Geometry check sheet. Reference: the model listing, model coordinates, mm. A direction names the side the tool comes from. Give positions to 0.01 mm unless a question says otherwise; leave off trailing zeros. Loops run counter-clockwise (first coordinate to the right, second up) from the corner with the lowest first, then second, coordinate; pieces in that order, holes last.
```python
from build123d import *

# Parameters (mm, degrees)
SKETCH_1_R          = 80
SKETCH_1_R_2        = 60
EXTRUDE_1_DEPTH     = 80
CUT_EXTRUDE_1_DEPTH = 139.564064606
CUT_EXTRUDE_2_DEPTH = 139.564064606
SKETCH_4_R          = 20
SKETCH_4_R_2        = 7.5
EXTRUDE_2_DEPTH     = 80
FILLET_1_R          = 10


with BuildPart() as part:
    # 草图1 → 凸台-拉伸1 (new body)
    with BuildSketch(Plane.XY):
        Circle(SKETCH_1_R)
        Circle(SKETCH_1_R_2, mode=Mode.SUBTRACT)
    extrude(amount=EXTRUDE_1_DEPTH)

    # 草图2 → 切除-拉伸1 (cut, through all)
    with BuildSketch(Plane.XY.offset(80)):
        Polygon((60.621778265, 30.265727793), (64.721778265, 32.632863896), (64.721778265, 37.367136104), (60.621778265, 39.734272207), (56.521778265, 37.367136104), (56.521778265, 32.632863896), align=None)
        Polygon((4.1, 67.632863896), (4.1, 72.367136104), (0, 74.734272207), (-4.1, 72.367136104), (-4.1, 67.632863896), (0, 65.265727793), align=None)
        Polygon((56.521778265, -37.367136104), (60.621778265, -39.734272207), (64.721778265, -37.367136104), (64.721778265, -32.632863896), (60.621778265, -30.265727793), (56.521778265, -32.632863896), align=None)
        Polygon((-4.1, -67.632863896), (-4.1, -72.367136104), (0, -74.734272207), (4.1, -72.367136104), (4.1, -67.632863896), (0, -65.265727793), align=None)
        Polygon((-60.621778265, -30.265727793), (-64.721778265, -32.632863896), (-64.721778265, -37.367136104), (-60.621778265, -39.734272207), (-56.521778265, -37.367136104), (-56.521778265, -32.632863896), align=None)
        Polygon((-56.521778265, 37.367136104), (-60.621778265, 39.734272207), (-64.721778265, 37.367136104), (-64.721778265, 32.632863896), (-60.621778265, 30.265727793), (-56.521778265, 32.632863896), align=None)
    extrude(amount=-CUT_EXTRUDE_1_DEPTH, mode=Mode.SUBTRACT)

    # 草图3 → 切除-拉伸2 (cut, through all)
    with BuildSketch(Plane.XY.offset(80)):
        with BuildLine():
            Line((0, 0), (-40, 69.282032303))
            ThreePointArc((-40, 69.282032303), (-40, -69.282032303), (80, 0))
            Line((80, 0), (0, 0))
        make_face()
    extrude(amount=-CUT_EXTRUDE_2_DEPTH, mode=Mode.SUBTRACT)

    # 草图4 → 凸台-拉伸2 (add)
    # profile 1 of 2: a face of its own
    with BuildSketch(Plane.XY.offset(80)):
        with Locations((0, 70)):
            Circle(SKETCH_4_R)
        with Locations((0, 70)):
            Circle(SKETCH_4_R_2, mode=Mode.SUBTRACT)
    # profile 2 of 2: a face of its own
    with BuildSketch(Plane.XY.offset(80)):
        with Locations((60.621778265, 35)):
            Circle(SKETCH_4_R)
        with Locations((60.621778265, 35)):
            Circle(SKETCH_4_R_2, mode=Mode.SUBTRACT)
    extrude(amount=-EXTRUDE_2_DEPTH)

    # 圆角1
    fillet_1_edges = [part.edges().sort_by_distance(p)[0] for p in [
        (76.622258716, 23.000640628, 40),
        (58.230268445, 54.856502229, 40),
        (18.391990271, 77.857142857, 40),
        (-18.391990271, 77.857142857, 40),
        (15.891853901, 57.857142857, 40),
        (-15.891853901, 57.857142857, 40),
        (58.051682455, 15.165822237, 40),
        (42.159828554, 42.69132062, 40),
    ]]
    fillet(fillet_1_edges, radius=FILLET_1_R)
    fillet_1_2_edges = [part.edges().sort_by_distance(p)[0] for p in [
        (60, 0, 40),
        (80, 0, 40),
        (-30, 51.961524227, 40),
        (-40, 69.282032303, 40),
    ]]
    fillet(fillet_1_2_edges, radius=FILLET_1_R - 0.0001)  # a hair under: the kernel refuses the full size


solid = part.part
```
1) Sectioned sample at A-A on y = 69. Enter the section's corners in (x, z), plus the area to 3 significant figures.
2) Depth check by flat-ended pin: P1, Ø8, axis at y = 34, z = 50.5, coming from the -X side; P2, Ø5, axis at y = 9, z = 22.5, coming from the +X side; P3, Ø6, axis at y = 71, z = 32.5, coming from the -X side. Enter the tip coordinate at first touch or a pass-through.
3) Sectioned sample at D-D on x = 44.5. Enter the section's corners in (y, z), plus the area to 3 significant figures.
4) Tool access check on faces 4 (the cylindrical face through (0, 50, 41)), 5 (the cylindrical face through (78.54, 15.22, 39.44)), 6 (the flat face through (2.02, 66.43, 40.56)). Record the directions out of +Z, -Z, +X, -X, +Y, -Y that give a thin tool (end or side, any length) a straight path to the whole face; none if there is none.
5) Sectioned sample at C-C on z = 63. Count the separate pieces of the cut face and the enclosed holes in it, plus the area to 3 significant figures.
6) Scan lines: line 1 along Y through (x, z) = (21, 57); line 2 along Y through (x, z) = (1, 62); line 3 along X through (y, z) = (84, 11). Record each from-to range of solid material in increasing order.
7) Sectioned sample at B-B on x = -6. Enter the section's corners in (y, z).
8) Mould release check, pull along Y, two halves, no side actions. Record for faces 1 (the cylindrical face through (-25.982, 75.663, 39.44)), 2 (the flat face through (26, 55, 0)), 3 (the flat face through (-2.02, 73.57, 40.56)): +Y half, -Y half, draft (parallel to the pull), parting line (faces both ways), or undercut.
Determined:
1. outline: (-35.15, 0) - (-4.1, 0) - (-4.1, 80) - (-35.15, 80) - close; (4.1, 0) - (40.48, 0) - (40.48, 80) - (4.1, 80) - close
1. area: 5,390 mm2
2. P1: stops at x = 40.62
2. P2: stops at x = 79.28
2. P3: stops at x = -35.52
3. outline: (23.16, 0) - (66.48, 0) - (66.48, 80) - (23.16, 80) - close
3. area: 3,470 mm2
4. face 4: +Z, -Z, -Y
4. face 5: +Z, -Z, +X
4. face 6: +Z, -Z
5. separate pieces: 1
5. enclosed holes: 2
5. area: 3,740 mm2
6. line 1: y = 56.13 to 77.31
6. line 2: y = 50.03 to 65.84, 74.16 to 89.97
6. line 3: x = -14.28 to 14.28
7. outline: (50.92, 0) - (89.08, 0) - (89.08, 80) - (50.92, 80) - close
8. face 1: +Y half
8. face 2: draft
8. face 3: undercut
